from build123d import *

# Parameters (mm, degrees)
ESQUISSE1_W                  = 40
ESQUISSE1_H                  = 5.5
BOSS_EXTRU_1_DEPTH           = 6
ESQUISSE2_R                  = 1.5
ENL_V_MAT_EXTRU_1_DEPTH      = 1
ENL_V_MAT_EXTRU_1_DEPTH_BACK = 7
ESQUISSE3_R                  = 1.65
ENL_V_MAT_EXTRU_2_DEPTH      = 1
ENL_V_MAT_EXTRU_2_DEPTH_BACK = 6.5


with BuildPart() as part:
    # Esquisse1 → Boss.-Extru.1 (new body)
    with BuildSketch(Plane.XY):
        with Locations((20, 2.75)):
            Rectangle(ESQUISSE1_W, ESQUISSE1_H)
    extrude(amount=BOSS_EXTRU_1_DEPTH)

    # Esquisse2 → Enlèv. mat.-Extru.1 (cut, two sides)
    with BuildSketch(Plane.XY.offset(6)) as enl_v_mat_extru_1_sk:
        with Locations((20, 2.75)):
            Circle(ESQUISSE2_R)
        with Locations((3, 2.75)):
            Circle(ESQUISSE2_R)
        with Locations((37, 2.75)):
            Circle(ESQUISSE2_R)
    extrude(amount=ENL_V_MAT_EXTRU_1_DEPTH, mode=Mode.SUBTRACT)
    extrude(enl_v_mat_extru_1_sk.sketch, amount=-ENL_V_MAT_EXTRU_1_DEPTH_BACK, mode=Mode.SUBTRACT)

    # Esquisse3 → Enlèv. mat.-Extru.2 (cut, two sides)
    with BuildSketch(Plane(origin=(0, 5.5, 0), x_dir=(1, 0, 0), z_dir=(0, 1, 0))) as enl_v_mat_extru_2_sk:
        with Locations((10, -3)):
            Circle(ESQUISSE3_R)
        with Locations((30, -3)):
            Circle(ESQUISSE3_R)
    extrude(amount=ENL_V_MAT_EXTRU_2_DEPTH, mode=Mode.SUBTRACT)
    extrude(enl_v_mat_extru_2_sk.sketch, amount=-ENL_V_MAT_EXTRU_2_DEPTH_BACK, mode=Mode.SUBTRACT)


solid = part.part
Here's how the part is built. I have some questions about the finished solid (model axes, mm). Give positions to 0.01 mm unless a question says otherwise; leave off trailing zeros. Write each loop counter-clockwise with the first axis right and the second up, starting at its lowest first coordinate (ties: lowest second). Pieces come first, ordered by that corner, then holes. Notation, with made-up numbers: (39.5, 65) -> (69.5, 65) arc R20 cw to (69.5, 99) -> close; hole circle Ø7 at (78.25, 88). An arc over 180 degrees is marked (long way). Use one line per item in the form item = value. Start each with the question number.
1. Imagine slicing it at A-A on y = 2.75. List the corners of the cut face in (x, z) for me.
2. Imagine slicing it at D-D on y = 0.85. List the corners of the cut face in (x, z) for me.
3. Thinking about a two-plate mould opening in Z: for faces 1 (the face through (20, 0, 3)), 2 (the face through (28.69, 2.79, 4)), 3 (the face through (20, 1, 0)), which applies, +Z half, -Z half, draft (parallel to the pull), parting line (faces both ways), or undercut?
4. If I drill on L1, parallel to X at y = 5.2, z = 3.1; L2, parallel to Y at x = 37, z = 3.75; L3, parallel to Z at x = 10, y = 1.3, over which ranges is the centre line in solid material (lowest first)?
5. Imagine slicing it at C-C on z = 2.15. List the corners of the cut face in (x, y) for me.
6. Will this pin go through, and if not, where does the flat tip stop? pin 1 Ø2.5 at (x, y) = (3, 2.75) entering from +Z.
7. Imagine slicing it at B-B on x = 20. List the corners of the cut face in (y, z) for me, plus the area to 3 significant figures.
Entries:
q1.outline = (0, 0) -> (1.5, 0) -> (1.5, 6) -> (0, 6) -> close; (4.5, 0) -> (18.5, 0) -> (18.5, 6) -> (4.5, 6) -> close; (21.5, 0) -> (35.5, 0) -> (35.5, 6) -> (21.5, 6) -> close; (38.5, 0) -> (40, 0) -> (40, 6) -> (38.5, 6) -> close; hole circle Ø3.3 at (10, 3); hole circle Ø3.3 at (30, 3)
q2.outline = (0, 0) -> (40, 0) -> (40, 6) -> (0, 6) -> close; hole circle Ø3.3 at (10, 3); hole circle Ø3.3 at (30, 3)
q3.face_1 = draft
q3.face_2 = undercut
q3.face_3 = -Z half
q4.L1 = 0 to 8.35, 11.65 to 28.35, 31.65 to 40
q4.L2 = 0 to 1.25, 4.25 to 5.5
q4.L3 = 0 to 1.35, 4.65 to 6
q5.outline = (0, 0) -> (8.59, 0) -> (8.59, 5.5) -> (0, 5.5) -> close; (11.41, 0) -> (28.59, 0) -> (28.59, 5.5) -> (11.41, 5.5) -> close; (31.41, 0) -> (40, 0) -> (40, 5.5) -> (31.41, 5.5) -> close; hole circle Ø3 at (3, 2.75); hole circle Ø3 at (20, 2.75); hole circle Ø3 at (37, 2.75)
q6.pin_1 = through
q7.outline = (0, 0) -> (1.25, 0) -> (1.25, 6) -> (0, 6) -> close; (4.25, 0) -> (5.5, 0) -> (5.5, 6) -> (4.25, 6) -> close
q7.area = 15.0 mm²
